Part model, mm, in its own coordinate system. A direction names the side the tool comes from. Coordinates: 2 decimals unless noted, no trailing zeros. Write each loop counter-clockwise with the first axis right and the second up, starting at its lowest first coordinate (ties: lowest second). Pieces come first, ordered by that corner, then holes. Notation, with made-up numbers: (49, 58) -> (79, 58) arc R17 cw to (79, 72) -> close; hole circle Ø6 at (79, -20). An arc over 180 degrees is marked (long way). Write item = value, one per line. Start each with the question number.
Q1. Band-saw the part on A-A, the plane y = 6. List the corners of the cut face in (x, z).
Q2. Pin check, flat tips, straight feed: P1, Ø0.6, axis at y = 49.5, z = 1, coming from the -X side; P2, Ø1, axis at x = 1.5, z = 1, coming from the -Y side; P3, Ø12, axis at x = 61, y = 46, coming from the -Z side; P4, Ø0.6, axis at x = 104.5, z = 0.5, coming from the +Y side. Stop position of each tip, or through.
Q3. Tool access for faces 1 (the flat face through (2, 16, 1)), 2 (the flat face through (2, 55, 1)), 3 (the flat face through (104, 9, 1)): list every direction of +Z, -Z, +X, -X, +Y, -Y with a clear straight run to the whole face (end or side of a thin tool).
Q4. Probe line 1 (X direction, y = 14, z = 1.1). List the from-to ranges inside material, lowest first.
Q5. Pull direction Y, two halves, no side cores. Call faces 4 (the flat face through (106, 10, 1)), 5 (the flat face through (102, 14, 1)), 6 (the flat face through (102, 50, 1)), 7 (the flat face through (52, 0, 1)): released by +Y, released by -Y, zero draft, split by the parting line, or undercut.
from build123d import *

# Parameters (mm, degrees)
SKETCH1_W           = 106
SKETCH1_H           = 64
BOSS_EXTRUDE1_DEPTH = 2
SKETCH2_W           = 4
SKETCH2_H           = 9
CUT_EXTRUDE1_DEPTH  = 124.838604643
CUT_EXTRUDE2_DEPTH  = 124.838604643


with BuildPart() as part:
    # Sketch1 → Boss-Extrude1 (new body)
    with BuildSketch(Plane.XY):
        with Locations((53, 32)):
            Rectangle(SKETCH1_W, SKETCH1_H)
    extrude(amount=BOSS_EXTRUDE1_DEPTH)

    # Sketch2 → Cut-Extrude1 (cut, through all)
    with BuildSketch(Plane.XY.offset(2)):
        with Locations((2, 59.5)):
            Rectangle(SKETCH2_W, SKETCH2_H)
        with Locations((2, 4.5)):
            Rectangle(SKETCH2_W, SKETCH2_H)
        with Locations((104, 4.5)):
            Rectangle(SKETCH2_W, SKETCH2_H)
        with Locations((104, 59.5)):
            Rectangle(SKETCH2_W, SKETCH2_H)
    extrude(amount=-CUT_EXTRUDE1_DEPTH, mode=Mode.SUBTRACT)

    # Sketch3 → Cut-Extrude2 (cut, through all)
    with BuildSketch(Plane.XY.offset(2)):
        with BuildLine():
            Line((106, 12), (103, 12))
            ThreePointArc((103, 12), (102.292893219, 12.292893219), (102, 13))
            Line((102, 13), (102, 15))
            ThreePointArc((102, 15), (102.292893219, 15.707106781), (103, 16))
            Line((103, 16), (106, 16))
            Line((106, 16), (106, 12))
        make_face()
        with BuildLine():
            Line((0, 12), (3, 12))
            ThreePointArc((3, 12), (3.707106781, 12.292893219), (4, 13))
            Line((4, 13), (4, 15))
            ThreePointArc((4, 15), (3.707106781, 15.707106781), (3, 16))
            Line((3, 16), (0, 16))
            Line((0, 16), (0, 12))
        make_face()
        with BuildLine():
            Line((0, 52), (3, 52))
            ThreePointArc((3, 52), (3.707106781, 51.707106781), (4, 51))
            Line((4, 51), (4, 49))
            ThreePointArc((4, 49), (3.707106781, 48.292893219), (3, 48))
            Line((3, 48), (0, 48))
            Line((0, 48), (0, 52))
        make_face()
        with BuildLine():
            Line((106, 52), (103, 52))
            ThreePointArc((103, 52), (102.292893219, 51.707106781), (102, 51))
            Line((102, 51), (102, 49))
            ThreePointArc((102, 49), (102.292893219, 48.292893219), (103, 48))
            Line((103, 48), (106, 48))
            Line((106, 48), (106, 52))
        make_face()
    extrude(amount=-CUT_EXTRUDE2_DEPTH, mode=Mode.SUBTRACT)


solid = part.part
Ans:
q1.outline = (4, 0) -> (102, 0) -> (102, 2) -> (4, 2) -> close
q2.P1 = 4
q2.P2 = 9
q2.P3 = 0
q2.P4 = 55
q3.face_1 = +Z, -Z, -X
q3.face_2 = +Z, -Z, -X, +Y
q3.face_3 = +Z, -Z, +X, -Y
q4.line_1 = 4 to 102
q5.face_4 = zero draft
q5.face_5 = undercut
q5.face_6 = undercut
q5.face_7 = released by -Y
